```python
from build123d import *
from OCP.BRepFilletAPI import BRepFilletAPI_MakeChamfer

# Parameters (mm, degrees)
EXTRUSION1_DEPTH           = 100
ESQUISSE2_R                = 1.5
EXTRUSION2_DEPTH           = 100
R_P_TITION_LIN_AIRE1_COUNT = 2
R_P_TITION_LIN_AIRE1_PITCH = 50
CHANFREIN1_SIZE            = 2.5
CHANFREIN3_SIZE            = 0.5
CHANFREIN3_SIZE2           = 0.353553391


with BuildPart() as part:
    # Esquisse1 → Extrusion1 (new body)
    with BuildSketch(Plane.XY):
        Polygon((0, 0), (1.5, 0), (15, 0), (15, 1.5), (1.5, 1.5), (1.5, 15), (0, 15), align=None)
    extrude(amount=EXTRUSION1_DEPTH)

    # Esquisse2 → Extrusion2 (cut)
    with BuildSketch(Plane.XZ):
        with Locations(Location((10, 75, 0), (0, 0, 270))):
            Circle(ESQUISSE2_R)
    extrusion2 = extrude(amount=-EXTRUSION2_DEPTH, mode=Mode.SUBTRACT)

    # Répétition linéaire1: Extrusion2 ×2
    with Locations(*[(0, 0, -i * R_P_TITION_LIN_AIRE1_PITCH) for i in range(1, R_P_TITION_LIN_AIRE1_COUNT)]):
        add(extrusion2, mode=Mode.SUBTRACT)

    # Chanfrein1
    chanfrein1_edges = [part.edges().sort_by_distance(p)[0] for p in [
        (0, 7.5, 100),
        (0, 7.5, 0),
    ]]
    chamfer(chanfrein1_edges, length=CHANFREIN1_SIZE)

    # Chanfrein3: one chamfer whose edges measure the first distance from different faces: ONE call of the kernel's chamfer builder (chamfer() names one face for all edges)
    chanfrein3_edges_1 = [part.edges().sort_by_distance(p)[0] for p in [
        (1.5, 8.25, 1),
    ]]
    chanfrein3_side_1 = [part.faces().sort_by_distance(p)[0] for p in [
        (0.828125, 7.078125, 1.671875),
    ]]
    chanfrein3_edges_2 = [part.edges().sort_by_distance(p)[0] for p in [
        (1.5, 8.25, 99),
    ]]
    chanfrein3_side_2 = [part.faces().sort_by_distance(p)[0] for p in [
        (0.828125, 7.078125, 98.328125),
    ]]
    chanfrein3 = BRepFilletAPI_MakeChamfer(part.part.solid().wrapped)
    for e in chanfrein3_edges_1:
        chanfrein3.Add(CHANFREIN3_SIZE, CHANFREIN3_SIZE2, e.wrapped, chanfrein3_side_1[0].wrapped)  # the first distance lies on this face
    for e in chanfrein3_edges_2:
        chanfrein3.Add(CHANFREIN3_SIZE, CHANFREIN3_SIZE2, e.wrapped, chanfrein3_side_2[0].wrapped)  # the first distance lies on this face
    add(Compound.cast(chanfrein3.Shape()), mode=Mode.REPLACE)


solid = part.part
```
Model file for the job. Use its own axes, mm. A direction names the side the tool comes from. Round coordinates to 2 decimals unless told otherwise and drop trailing zeros. Write each loop counter-clockwise with the first axis right and the second up, starting at its lowest first coordinate (ties: lowest second). Pieces come first, ordered by that corner, then holes. Notation, with made-up numbers: (30.25, 65) - (67.25, 65) arc R21 cw to (67.25, 81) - close; hole circle Ø6 at (-17, 6). An arc over 180 degrees is marked (long way). One line per item, written item: value.
(1) Two-plate mould, pull along X, no slides. Class faces 3 (the cylindrical face through (10.45, 0.74, 73.57)), 4 (the flat face through (7, 0, 49)), 5 (the flat face through (0.7, 7.6, 1.8)): pulls with the +X half, pulls with the -X half, needs draft (parallel to the pull), parting line crosses it, or undercut.
Values follow:
face 3: undercut
face 4: needs draft
face 5: pulls with the -X half
(2) Drop flat-ended pins along their axis: P1, Ø5, axis at x = 6, z = 45, coming from the -Y side; P2, Ø6, axis at y = 12, z = 46, coming from the +X side. Give the stop position or say it passes through.
Values follow:
P1: stops at y = 0
P2: stops at x = 1.5
(3) Wall check: probe 1 along X at (y, z) = (0.8, 75); probe 2 along Y at (x, z) = (6, 52). Give the ranges that are in metal, low to high.
Values follow:
probe 1: x = 0 to 8.5, 11.5 to 15
probe 2: y = 0 to 1.5
(4) Cut at A-A, the plane z = 75. Give the cut face in (x, y), plus the area to 4 significant figures.
Values follow:
outline: (0, 0) - (8.5, 0) - (8.5, 1.5) - (1.5, 1.5) - (1.5, 15) - (0, 15) - close; (11.5, 0) - (15, 0) - (15, 1.5) - (11.5, 1.5) - close
area: 38.25 mm²
(5) Cut at D-D, the plane y = 5.5. Give the cut face in (x, z), plus the area to 3 significant figures.
Values follow:
outline: (0, 2.5) - (1.15, 1.35) - (1.5, 1.35) - (1.5, 98.65) - (1.15, 98.65) - (0, 97.5) - close
area: 145 mm²
(6) Cut at B-B, the plane x = 10. Give the cut face in (y, z), plus the area to 3 significant figures.
Values follow:
outline: (0, 0) - (1.5, 0) - (1.5, 23.5) - (0, 23.5) - close; (0, 26.5) - (1.5, 26.5) - (1.5, 73.5) - (0, 73.5) - close; (0, 76.5) - (1.5, 76.5) - (1.5, 100) - (0, 100) - close
area: 141 mm²
(7) Cut at C-C, the plane z = 30.5. Give the cut face in (x, y), plus the area to 4 significant figures.
Values follow:
outline: (0, 0) - (15, 0) - (15, 1.5) - (1.5, 1.5) - (1.5, 15) - (0, 15) - close
area: 42.75 mm²
(8) 3-axis set-ups, long thin cutter, end or side, ignore diameter. For faces 1 (the flat face through (1.5, 8, 49)), 2 (the cylindrical face through (9.1, 0.7, 26.2)): which of +Z, -Z, +X, -X, +Y, -Y reach the whole face in a straight line?
Values follow:
face 1: +Z, -Z, +X, +Y
face 2: +Y, -Y
